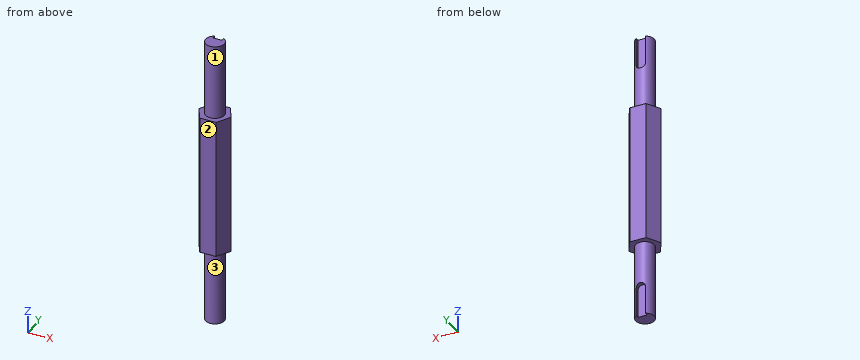
```python
from build123d import *

# Parameters (mm, degrees)
BOSS_EXTRUDE1_DEPTH  = 75
SKETCH2_R            = 10
BOSS_EXTRUDE2_DEPTH  = 80
BOSS_EXTRUDE3_START  = 80
SKETCH3_R            = 10
BOSS_EXTRUDE3_DEPTH  = 80
SKETCH4_W            = 10
SKETCH4_H            = 18.646809019
CUT_EXTRUDE1_DEPTH   = 35
FILLET1_R            = 5
FILLET1_OF_MIRROR1_R = 5


with BuildPart() as part:
    # Sketch1 → Boss-Extrude1 (new, symmetric)
    with BuildSketch(Plane.XY):
        Polygon((8.660254038, 15), (-8.660254038, 15), (-17.320508076, 0), (-8.660254038, -15), (8.660254038, -15), (17.320508076, 0), align=None)
    extrude(amount=BOSS_EXTRUDE1_DEPTH, both=True)

    # Sketch2 → Boss-Extrude2 (add)
    with BuildSketch(Plane.XY.offset(75)):
        Circle(SKETCH2_R)
    extrude(amount=BOSS_EXTRUDE2_DEPTH)

    # Sketch3 → Boss-Extrude3 (add)
    with BuildSketch(Plane(origin=(0, 0, -75), x_dir=(-1, 0, 0), z_dir=(0, 0, -1)).offset(BOSS_EXTRUDE3_START)):
        with Locations(Location((0, 0, 0), (0, 0, 180))):
            Circle(SKETCH3_R)
    extrude(amount=-BOSS_EXTRUDE3_DEPTH)

    # Sketch4 → Cut-Extrude1 (cut)
    with BuildSketch(Plane.XY.offset(155)):
        with Locations((0, 14.32340451)):
            Rectangle(SKETCH4_W, SKETCH4_H)
    cut_extrude1 = extrude(amount=-CUT_EXTRUDE1_DEPTH, mode=Mode.SUBTRACT)

    # Fillet1
    fillet1_edges = [part.edges().sort_by_distance(p)[0] for p in [
        (5, 6.830127019, 120),
        (-5, 6.830127019, 120),
    ]]
    fillet(fillet1_edges, radius=FILLET1_R - 0.0001)  # a hair under: the kernel refuses the full size

    # Mirror1: Cut-Extrude1 across plane
    add(cut_extrude1.mirror(Plane.XY), mode=Mode.SUBTRACT)

    # Fillet1 of Mirror1
    fillet1_of_mirror1_edges = [part.edges().sort_by_distance(p)[0] for p in [
        (5, 6.830127019, -120),
        (-5, 6.830127019, -120),
    ]]
    fillet(fillet1_of_mirror1_edges, radius=FILLET1_OF_MIRROR1_R - 0.0001)  # a hair under: the kernel refuses the full size


solid = part.part
```
Here's how the part is built. I have some questions about the finished solid (model axes, mm). Face numbers are marked on the shaded views. A direction names the side the tool comes from. Give positions to 0.01 mm unless a question says otherwise; leave off trailing zeros. Write each question's results on one line, items separated by ' | '.
Item 1: If I drill on L1, parallel to Z at x = -11.5, y = 3.25; L2, parallel to X at y = -4.5, z = -31.5; L3, parallel to Y at x = 14.5, z = 47, over which ranges is the centre line in solid material (lowest first)?
Output:
L1: z = -75 to 75 | L2: x = -14.72 to 14.72 | L3: y = -4.89 to 4.89
Item 2: For pin 1 Ø1.1 at (y, z) = (7, 142) entering from +X; pin 2 Ø1 at (x, y) = (-13.5, 9) entering from +Z; pin 3 Ø3 at (y, z) = (6.5, 138.5) entering from -X; pin 4 Ø5 at (x, z) = (-2, -134) entering from +Y, each with a flat end and sliding along its axis, tell me the tip position at first contact or that it passes through.
Output:
pin 1: stops at x = 7.64 | pin 2: passes through | pin 3: stops at x = -8.66 | pin 4: stops at y = 5
Item 3: On a 3-axis mill with a long thin cutter (end or side, diameter ignored), from which of +Z, -Z, +X, -X, +Y, -Y can I reach the whole of each face in a straight line? I mean the marked faces 1, 2 and 3. Say none if no direction works.
Output:
face 1: +Z | face 2: +Z, -Z, +X, -X, -Y | face 3: -Z
